Input: part model. Units: mm. Frame: model coordinates. Round coordinates to 2 decimals unless told otherwise and drop trailing zeros. Loops run counter-clockwise (first coordinate to the right, second up) from the corner with the lowest first, then second, coordinate; pieces in that order, holes last.
(1) Draft query along Y for faces 1 (the face through (64, 41.612, 151)), 2 (the face through (64, -59.534, 151)), 3 (the face through (10.025, -50, 151)), 4 (the face through (35.004, -8.117, 150.81)). Return one class per face: released by +Y, released by -Y, zero draft, split by the parting line, or undercut.
(2) First-contact query: pin 1 Ø12 at (y, z) = (-23, 144.5) entering from -X. Flat tip, straight axial feed; report the tip coordinate or a pass-through.
(3) Cut plane A-A, the plane x = 26. Output: boundary loops of the cut face in (y, z), and give its area (3 significant figures).
(4) Cut plane B-B, the plane z = 136.5. Output: boundary loops of the cut face in (x, y).
(5) Line query: line 1 (Y direction, x = 15, z = 224.5); line 2 (Y direction, x = 30, z = 98); line 3 (X direction, y = -32, z = 114). Output: solid intervals per line, ascending.
from build123d import *

# Parameters (mm, degrees)
SKETCH017_W          = 108.598946
SKETCH017_H          = 101.145454
PAD007_DEPTH         = 170
SKETCH018_R          = 35
POCKET011_DEPTH      = 0.001
POCKET012_DEPTH      = 0.001
POCKET012_DEPTH_BACK = 170.001


with BuildPart() as part:
    # Sketch017 → Pad007 (new body)
    with BuildSketch(Plane.XY):
        with Locations((64.32481, -8.960884)):
            Rectangle(SKETCH017_W, SKETCH017_H)
    extrude(amount=PAD007_DEPTH)

    # Sketch018 → Pocket011 (cut, through all)
    with BuildSketch(Plane.XY):
        with Locations((0.01, -7.49)):
            Circle(SKETCH018_R)
    extrude(amount=-POCKET011_DEPTH, mode=Mode.SUBTRACT)

    # Sketch018 → Pocket012 (cut, two sides)
    with BuildSketch(Plane.XY) as pocket012_sk:
        with Locations((0.01, -7.49)):
            Circle(SKETCH018_R)
    extrude(amount=-POCKET012_DEPTH, mode=Mode.SUBTRACT)
    extrude(pocket012_sk.sketch, amount=POCKET012_DEPTH_BACK, mode=Mode.SUBTRACT)


with BuildPart() as part_1:
    # Body005 placement: moved
    add(part.part.moved(Location((0, 0, 67))))


solid = part_1.part
Reported:
1. face 1: released by +Y
1. face 2: released by -Y
1. face 3: zero draft
1. face 4: undercut
2. pin 1: stops at x = 27.62
3. outline: (-59.53, 67) - (-30.93, 67) - (-30.93, 237) - (-59.53, 237) - close; (15.95, 67) - (41.61, 67) - (41.61, 237) - (15.95, 237) - close
3. area: 9,220 mm2
4. outline: (10.03, -59.53) - (118.62, -59.53) - (118.62, 41.61) - (10.03, 41.61) - (10.03, 26.05) arc R35 cw to (10.03, -41.03) - close
5. line 1: y = -59.53 to -39.12, 24.14 to 41.61
5. line 2: y = -59.53 to -25.53, 10.55 to 41.61
5. line 3: x = 25 to 118.62
